from build123d import *

# Parameters (mm, degrees)
SKETCH1_R           = 85
SKETCH1_R_2         = 75
BOSS_EXTRUDE1_DEPTH = 35
SKETCH2_R           = 85
BOSS_EXTRUDE2_DEPTH = 4
SKETCH3_R           = 5
BOSS_EXTRUDE3_DEPTH = 32.5
SKETCH4_R           = 95.738737625
SKETCH4_R_2         = 85
CUT_EXTRUDE1_DEPTH  = 67
CUT_EXTRUDE2_DEPTH  = 58
SKETCH6_R           = 85
SKETCH6_R_2         = 75
BOSS_EXTRUDE4_DEPTH = 28


with BuildPart() as part:
    # Sketch1 → Boss-Extrude1 (new body)
    with BuildSketch(Plane(origin=(0, 0, 0), x_dir=(1, 0, 0), z_dir=(0, 1, 0))):
        Circle(SKETCH1_R)
        Circle(SKETCH1_R_2, mode=Mode.SUBTRACT)
    extrude(amount=BOSS_EXTRUDE1_DEPTH)

    # Sketch2 → Boss-Extrude2 (add)
    with BuildSketch(Plane(origin=(0, 35, 0), x_dir=(1, 0, 0), z_dir=(0, 1, 0))):
        Circle(SKETCH2_R)
    extrude(amount=BOSS_EXTRUDE2_DEPTH)

    # Sketch3 → Boss-Extrude3 (add, symmetric)
    with BuildSketch(Plane.XY):
        with BuildLine():
            Line((-85, 39), (-61.181000395, 88.51271152))
            ThreePointArc((-61.181000395, 88.51271152), (0, 126.386849251), (61.181000395, 88.51271152))
            Line((61.181000395, 88.51271152), (85, 39))
            Line((85, 39), (-85, 39))
        make_face()
        with Locations((0, 81.844221237)):
            Circle(SKETCH3_R, mode=Mode.SUBTRACT)
    extrude(amount=BOSS_EXTRUDE3_DEPTH, both=True)

    # Sketch4 → Cut-Extrude1 (cut)
    with BuildSketch(Plane(origin=(0, 39, 0), x_dir=(1, 0, 0), z_dir=(0, 1, 0))):
        Circle(SKETCH4_R)
        Circle(SKETCH4_R_2, mode=Mode.SUBTRACT)
    extrude(amount=CUT_EXTRUDE1_DEPTH, mode=Mode.SUBTRACT)

    # Sketch5 → Cut-Extrude2 (cut)
    with BuildSketch(Plane.XZ.offset(-35)):
        with BuildLine():
            Line((-15.1, -17.6), (15.1, -17.6))
            ThreePointArc((15.1, -17.6), (16.867766953, -16.867766953), (17.6, -15.1))
            Line((17.6, -15.1), (17.6, 15.1))
            ThreePointArc((17.6, 15.1), (16.867766953, 16.867766953), (15.1, 17.6))
            Line((15.1, 17.6), (-15.1, 17.6))
            ThreePointArc((-15.1, 17.6), (-16.867766953, 16.867766953), (-17.6, 15.1))
            Line((-17.6, 15.1), (-17.6, -15.1))
            ThreePointArc((-17.6, -15.1), (-16.867766953, -16.867766953), (-15.1, -17.6))
        make_face()
    extrude(amount=-CUT_EXTRUDE2_DEPTH, mode=Mode.SUBTRACT)

    # Sketch6 → Boss-Extrude4 (add)
    with BuildSketch(Plane.XZ):
        Circle(SKETCH6_R)
        Circle(SKETCH6_R_2, mode=Mode.SUBTRACT)
    extrude(amount=BOSS_EXTRUDE4_DEPTH)


solid = part.part
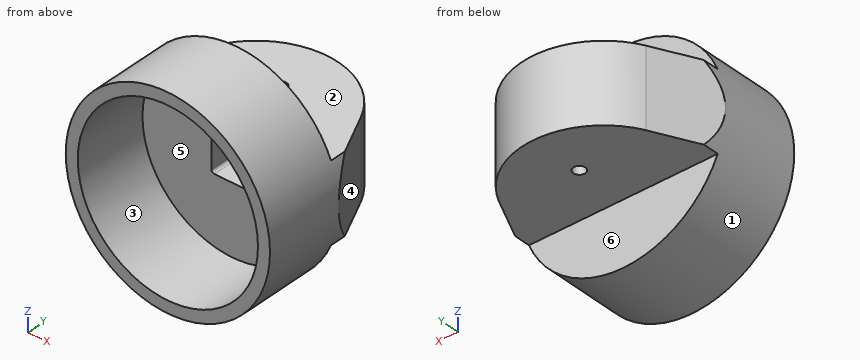
The model under review builds one solid part; all positions refer to its coordinate system, in mm. Face numbers are marked on the shaded views. A direction names the side the tool comes from. Give positions to 0.01 mm unless a question says otherwise; leave off trailing zeros. Loops run counter-clockwise (first coordinate to the right, second up) from the corner with the lowest first, then second, coordinate; pieces in that order, holes last. Notation, with made-up numbers: (40.5, 10) -> (64.5, 10) arc R8 cw to (64.5, 25) -> close; hole circle Ø8 at (-28, -24). An arc over 180 degrees is marked (long way). Answer as a JSON object with one key per item and string values. Group by question number.
Q1. Take a section at C-C (y = -18). Write out the cut boundary in (x, z).
Q2. Wall thickness on line 1 along Z through (x, y) = (0, 8); line 2 along Z through (x, y) = (29, 113): over which ranges is each line inside the solid? List them lowest first.
Q3. Tool access review of the marked faces 4, 5 and 6: name each direction out of +Z, -Z, +X, -X, +Y, -Y from which nothing blocks a thin tool from reaching the whole face with its end or side.
Q4. Take a section at D-D (x = 31). Write out the cut boundary in (y, z).
Q5. Insertion check: pin 1 (8 mm diameter, centred on x = -16.5, y = 25, fed in from +Z); pin 2 (4 mm diameter, centred on x = 60.5, z = 28.5, fed in from +Y); pin 3 (9 mm diameter, centred on y = 71.5, z = -2, fed in from -X). Each pin has a flat end and moves straight along its axis. Give the tip position at first contact, or say it passes through.
Q6. Draft analysis for pull direction X (two halves, no side actions). For the marked faces 1, 2 and 3, state which applies: pulls with the +X half, pulls with the -X half, needs draft (parallel to the pull), parting line crosses it, or undercut.
Q7. Take a section at B-B (z = 0). Write out the cut boundary in (x, y), plus the area to 3 significant figures.
Q8. Take a section at A-A (x = 0). Write out the cut boundary in (y, z), plus the area to 3 significant figures.
Answer below:
{
 "1": {"outline": "circle Ø170 at (0, 0); hole circle Ø150 at (0, 0)"},
 "2": {"line 1": "z = -85 to -75, 75 to 85", "line 2": "z = -32.5 to 32.5"},
 "3": {"face 4": "+Z, -Z, +X, +Y", "face 5": "-Y", "face 6": "-Z, +X, -X, +Y"},
 "4": {"outline": "(-28, -79.15) -> (39, -79.15) -> (39, -32.5) -> (118.95, -32.5) -> (118.95, 32.5) -> (39, 32.5) -> (39, 79.15) -> (-28, 79.15) -> (-28, 68.29) -> (35, 68.29) -> (35, -68.29) -> (-28, -68.29) -> close"},
 "5": {"pin 1": "stops at z = 84.08", "pin 2": "stops at y = 93.39", "pin 3": "stops at x = -71.53"},
 "6": {"face 1": "parting line crosses it", "face 2": "needs draft", "face 3": "undercut"},
 "7": {"outline": "(-85, -28) -> (-75, -28) -> (-75, 35) -> (-17.6, 35) -> (-17.6, 93) -> (17.6, 93) -> (17.6, 35) -> (75, 35) -> (75, -28) -> (85, -28) -> (85, 39) -> (61.18, 88.51) arc R68.35 ccw to (-61.18, 88.51) -> (-85, 39) -> close", "area": "10,500 mm2"},
 "8": {"outline": "(-28, -85) -> (39, -85) -> (39, -32.5) -> (76.84, -32.5) -> (76.84, -17.6) -> (35, -17.6) -> (35, -75) -> (-28, -75) -> close; (-28, 75) -> (35, 75) -> (35, 17.6) -> (76.84, 17.6) -> (76.84, 32.5) -> (39, 32.5) -> (39, 85) -> (-28, 85) -> close; (86.84, -32.5) -> (126.39, -32.5) -> (126.39, 32.5) -> (86.84, 32.5) -> (86.84, 17.6) -> (93, 17.6) -> (93, -17.6) -> (86.84, -17.6) -> close", "area": "5,280 mm2"}
}
